Check sheet for the modelled part. Datum: model origin and axes. Units: mm. Round coordinates to 2 decimals unless told otherwise and drop trailing zeros. Order: outer loops, then holes, each group sorted by start corner. A loop starts at its lowest first (then second) coordinate and runs counter-clockwise, first axis right, second up. Notation, with made-up numbers: (52.25, -12.75) -> (56.25, -12.75) arc R19 cw to (56.25, 7.25) -> close; hole circle Ø6 at (-21.5, 58.5). An arc over 180 degrees is marked (long way). Answer in a Markdown table with one row per item.
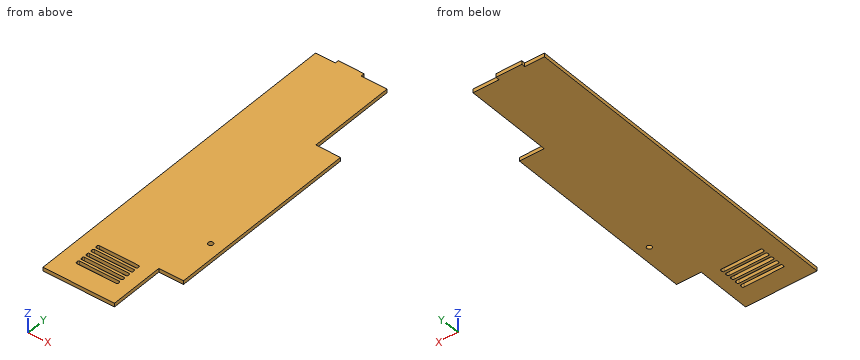
from build123d import *

# Parameters (mm, degrees)
SKETCH1_R           = 2
BOSS_EXTRUDE1_DEPTH = 3


with BuildPart() as part:
    # Sketch1 → Boss-Extrude1 (new body)
    with BuildSketch(Plane.XY):
        Polygon((18, -23.070954543), (18, 48.929045457), (-3, 48.929045457), (-3, 51.929045457), (-24, 51.929045457), (-24, 48.929045457), (-40, 48.929045457), (-40, -227.070954543), (18, -227.070954543), (18, -182.070954543), (38, -182.070954543), (38, -23.070954543), align=None)
        with BuildLine():
            Line((-25.70047512, -207.785634012), (6.29952488, -207.785634012))
            ThreePointArc((6.29952488, -207.785634012), (7.006631662, -208.078527231), (7.29952488, -208.785634012))
            Line((7.29952488, -208.785634012), (7.29952488, -209.785634012))
            ThreePointArc((7.29952488, -209.785634012), (7.006631662, -210.492740793), (6.29952488, -210.785634012))
            Line((6.29952488, -210.785634012), (-25.70047512, -210.785634012))
            ThreePointArc((-25.70047512, -210.785634012), (-26.407581901, -210.492740793), (-26.70047512, -209.785634012))
            Line((-26.70047512, -209.785634012), (-26.70047512, -208.785634012))
            ThreePointArc((-26.70047512, -208.785634012), (-26.407581901, -208.078527231), (-25.70047512, -207.785634012))
        make_face(mode=Mode.SUBTRACT)
        with BuildLine():
            Line((-25.70047512, -202.785634012), (6.29952488, -202.785634012))
            ThreePointArc((6.29952488, -202.785634012), (7.006631662, -203.078527231), (7.29952488, -203.785634012))
            Line((7.29952488, -203.785634012), (7.29952488, -204.785634012))
            ThreePointArc((7.29952488, -204.785634012), (7.006631662, -205.492740793), (6.29952488, -205.785634012))
            Line((6.29952488, -205.785634012), (-25.70047512, -205.785634012))
            ThreePointArc((-25.70047512, -205.785634012), (-26.407581901, -205.492740793), (-26.70047512, -204.785634012))
            Line((-26.70047512, -204.785634012), (-26.70047512, -203.785634012))
            ThreePointArc((-26.70047512, -203.785634012), (-26.407581901, -203.078527231), (-25.70047512, -202.785634012))
        make_face(mode=Mode.SUBTRACT)
        with BuildLine():
            Line((-25.70047512, -197.785634012), (6.29952488, -197.785634012))
            ThreePointArc((6.29952488, -197.785634012), (7.006631662, -198.078527231), (7.29952488, -198.785634012))
            Line((7.29952488, -198.785634012), (7.29952488, -199.785634012))
            ThreePointArc((7.29952488, -199.785634012), (7.006631662, -200.492740793), (6.29952488, -200.785634012))
            Line((6.29952488, -200.785634012), (-25.70047512, -200.785634012))
            ThreePointArc((-25.70047512, -200.785634012), (-26.407581901, -200.492740793), (-26.70047512, -199.785634012))
            Line((-26.70047512, -199.785634012), (-26.70047512, -198.785634012))
            ThreePointArc((-26.70047512, -198.785634012), (-26.407581901, -198.078527231), (-25.70047512, -197.785634012))
        make_face(mode=Mode.SUBTRACT)
        with BuildLine():
            Line((-25.70047512, -192.785634012), (6.29952488, -192.785634012))
            ThreePointArc((6.29952488, -192.785634012), (7.006631662, -193.078527231), (7.29952488, -193.785634012))
            Line((7.29952488, -193.785634012), (7.29952488, -194.785634012))
            ThreePointArc((7.29952488, -194.785634012), (7.006631662, -195.492740793), (6.29952488, -195.785634012))
            Line((6.29952488, -195.785634012), (-25.70047512, -195.785634012))
            ThreePointArc((-25.70047512, -195.785634012), (-26.407581901, -195.492740793), (-26.70047512, -194.785634012))
            Line((-26.70047512, -194.785634012), (-26.70047512, -193.785634012))
            ThreePointArc((-26.70047512, -193.785634012), (-26.407581901, -193.078527231), (-25.70047512, -192.785634012))
        make_face(mode=Mode.SUBTRACT)
        with BuildLine():
            Line((-25.70047512, -187.785634012), (6.29952488, -187.785634012))
            ThreePointArc((6.29952488, -187.785634012), (7.006631662, -188.078527231), (7.29952488, -188.785634012))
            Line((7.29952488, -188.785634012), (7.29952488, -189.785634012))
            ThreePointArc((7.29952488, -189.785634012), (7.006631662, -190.492740793), (6.29952488, -190.785634012))
            Line((6.29952488, -190.785634012), (-25.70047512, -190.785634012))
            ThreePointArc((-25.70047512, -190.785634012), (-26.407581901, -190.492740793), (-26.70047512, -189.785634012))
            Line((-26.70047512, -189.785634012), (-26.70047512, -188.785634012))
            ThreePointArc((-26.70047512, -188.785634012), (-26.407581901, -188.078527231), (-25.70047512, -187.785634012))
        make_face(mode=Mode.SUBTRACT)
        with Locations((28, -142.070954543)):
            Circle(SKETCH1_R, mode=Mode.SUBTRACT)
    extrude(amount=BOSS_EXTRUDE1_DEPTH)


solid = part.part
Item 1: Cross-section at A-A (x = 3.5). Record the boundary of the cut face in (y, z).
Result sheet:
| item | result |
|---|---|
| outline | (-227.07, 0) -> (-210.79, 0) -> (-210.79, 3) -> (-227.07, 3) -> close; (-207.79, 0) -> (-205.79, 0) -> (-205.79, 3) -> (-207.79, 3) -> close; (-202.79, 0) -> (-200.79, 0) -> (-200.79, 3) -> (-202.79, 3) -> close; (-197.79, 0) -> (-195.79, 0) -> (-195.79, 3) -> (-197.79, 3) -> close; (-192.79, 0) -> (-190.79, 0) -> (-190.79, 3) -> (-192.79, 3) -> close; (-187.79, 0) -> (48.93, 0) -> (48.93, 3) -> (-187.79, 3) -> close |
Item 2: Depth check by flat-ended pin: P1, Ø0.9, axis at x = 10.5, z = 1, coming from the +Y side; P2, Ø0.5, axis at y = -204.5, z = 2, coming from the +X side. Enter the tip coordinate at first touch or a pass-through.
Result sheet:
| item | result |
|---|---|
| P1 | stops at y = 48.93 |
| P2 | stops at x = 18 |
Item 3: Cross-section at D-D (z = 2.05). State how many separate pieces and enclosed holes the cut face has, and give its area (3 significant figures).
Result sheet:
| item | result |
|---|---|
| separate pieces | 1 |
| enclosed holes | 6 |
| area | 18,700 mm^2 |
Item 4: Cross-section at C-C (y = 17). Record the boundary of the cut face in (x, z).
Result sheet:
| item | result |
|---|---|
| outline | (-40, 0) -> (18, 0) -> (18, 3) -> (-40, 3) -> close |
Item 5: Scan lines: line 1 (Y direction, x = -17, z = 1.5); line 2 (Y direction, x = 28, z = 1.4); line 3 (Y direction, x = 16, z = 1.95). Record each from-to range of solid material in increasing order. Write a range as [from, to].
Result sheet:
| item | result |
|---|---|
| line 1 | y = [-227.07, -210.79], [-207.79, -205.79], [-202.79, -200.79], [-197.79, -195.79], [-192.79, -190.79], [-187.79, 51.93] |
| line 2 | y = [-182.07, -144.07], [-140.07, -23.07] |
| line 3 | y = [-227.07, 48.93] |
Item 6: Cross-section at B-B (x = -14). Record the boundary of the cut face in (y, z).
Result sheet:
| item | result |
|---|---|
| outline | (-227.07, 0) -> (-210.79, 0) -> (-210.79, 3) -> (-227.07, 3) -> close; (-207.79, 0) -> (-205.79, 0) -> (-205.79, 3) -> (-207.79, 3) -> close; (-202.79, 0) -> (-200.79, 0) -> (-200.79, 3) -> (-202.79, 3) -> close; (-197.79, 0) -> (-195.79, 0) -> (-195.79, 3) -> (-197.79, 3) -> close; (-192.79, 0) -> (-190.79, 0) -> (-190.79, 3) -> (-192.79, 3) -> close; (-187.79, 0) -> (51.93, 0) -> (51.93, 3) -> (-187.79, 3) -> close |
